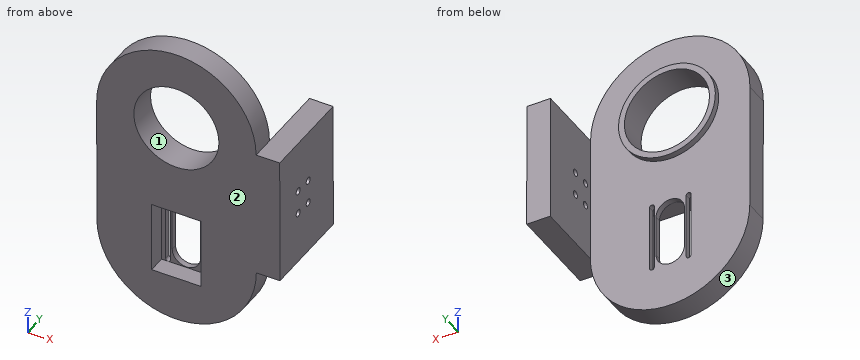
```python
from build123d import *

# Parameters (mm, degrees)
BOSS_EXTRUDE1_DEPTH = 20
SKETCH8_W           = 42
SKETCH8_H           = 60
CUT_EXTRUDE1_DEPTH  = 15
CUT_EXTRUDE2_START  = -5
CUT_EXTRUDE2_DEPTH  = 5
SKETCH10_R          = 36
CUT_EXTRUDE3_DEPTH  = 159.272933389
SKETCH11_R          = 41
SKETCH11_R_2        = 36
BOSS_EXTRUDE4_DEPTH = 5
SKETCH2_W           = 108.361469825
SKETCH2_H           = 80
SKETCH2_R           = 3
BOSS_EXTRUDE6_DEPTH = 20


# Read off the part's stored shape, not the designer's step: Cut-Extrude2
with BuildPart() as part:
    # Sketch1 → Boss-Extrude1 (new body)
    with BuildSketch(Plane(origin=(0, 0, 0), x_dir=(1, 0, 0), z_dir=(0, 1, 0))):
        with BuildLine():
            Line((47.685345344, 62.745795153), (47.499901156, -45.615515992))
            ThreePointArc((47.499901156, -45.615515992), (-20.115515992, -112.999901156), (-87.499901156, -45.384484008))
            Line((-87.499901156, -45.384484008), (-87.314456968, 62.976827137))
            ThreePointArc((-87.314456968, 62.976827137), (-19.69903982, 130.361212301), (47.685345344, 62.745795153))
        make_face()
    extrude(amount=BOSS_EXTRUDE1_DEPTH)

    # Sketch8 → Cut-Extrude1 (cut)
    with BuildSketch(Plane.XZ):
        with Locations((-20, -62.5)):
            Rectangle(SKETCH8_W, SKETCH8_H)
    extrude(amount=-CUT_EXTRUDE1_DEPTH, mode=Mode.SUBTRACT)

    # Cut-Extrude2 outline → Cut-Extrude2 (cut)
    with BuildSketch(Plane.XZ.offset(-15).offset(CUT_EXTRUDE2_START)):
        with BuildLine():
            Line((-6.5, -34.5), (-6.5, -90.5))
            ThreePointArc((-6.5, -90.5), (-4.5, -92.5), (-2.5, -90.5))
            Line((-2.5, -90.5), (-2.5, -34.5))
            ThreePointArc((-2.5, -34.5), (-4.5, -32.5), (-6.5, -34.5))
        make_face()
        with BuildLine():
            ThreePointArc((-8, -45), (-20, -33), (-32, -45))
            Line((-32, -45), (-32, -80))
            ThreePointArc((-32, -80), (-20, -92), (-8, -80))
            Line((-8, -80), (-8, -45))
        make_face()
        with BuildLine():
            Line((-37.5, -34.5), (-37.5, -90.5))
            ThreePointArc((-37.5, -90.5), (-35.5, -92.5), (-33.5, -90.5))
            Line((-33.5, -90.5), (-33.5, -34.5))
            ThreePointArc((-33.5, -34.5), (-35.5, -32.5), (-37.5, -34.5))
        make_face()
    extrude(amount=CUT_EXTRUDE2_DEPTH, mode=Mode.SUBTRACT)

    # Sketch10 → Cut-Extrude3 (cut, through all)
    with BuildSketch(Plane.XZ):
        with Locations(Location((-20, 45.5, 0), (0, 0, 270))):
            Circle(SKETCH10_R)
    extrude(amount=-CUT_EXTRUDE3_DEPTH, mode=Mode.SUBTRACT)

    # Sketch11 → Boss-Extrude4 (add)
    with BuildSketch(Plane(origin=(0, 20, 0), x_dir=(1, 0, 0), z_dir=(0, 1, 0))):
        with Locations(Location((-20, -45.5, 0), (0, 0, 270))):
            Circle(SKETCH11_R)
        with Locations(Location((-20, -45.5, 0), (0, 0, 90))):
            Circle(SKETCH11_R_2, mode=Mode.SUBTRACT)
    extrude(amount=BOSS_EXTRUDE4_DEPTH)

    # Sketch2 → Boss-Extrude6 (add)
    with BuildSketch(Plane(origin=(47.577825951, 0, 0.081422338), x_dir=(0.0017113480294572096, 0, -0.9999985356428889), z_dir=(0.999998535642889, 0, 0.0017113480294572096))):
        with Locations((8.64657458, 40)):
            Rectangle(SKETCH2_W, SKETCH2_H)
        with Locations((-1.551375347, 27.5)):
            Circle(SKETCH2_R, mode=Mode.SUBTRACT)
        with Locations((18.448624653, 27.5)):
            Circle(SKETCH2_R, mode=Mode.SUBTRACT)
        with Locations((18.448624653, 42.5)):
            Circle(SKETCH2_R, mode=Mode.SUBTRACT)
        with Locations((-1.551375347, 42.5)):
            Circle(SKETCH2_R, mode=Mode.SUBTRACT)
    extrude(amount=BOSS_EXTRUDE6_DEPTH)


solid = part.part
```
Could you check a few things on this model? Use its own coordinates, in mm. Face numbers are marked on the shaded views. Coordinates: 2 decimals unless noted, no trailing zeros. Order: outer loops, then holes, each group sorted by start corner. A loop starts at its lowest first (then second) coordinate and runs counter-clockwise, first axis right, second up. Notation, with made-up numbers: M 37.5,-22 L 81.5,-22 A6 cw 81.5,-16 Z; hole C 76.25,25 d2. An arc over 180 degrees is marked long. Use one line per item in the form item = value. Start each with the question number.
1. Please list where these lines run through material, in increasing order: line 1 (Z direction, x = -20, y = 11); line 2 (Z direction, x = 57, y = 28); line 3 (X direction, y = 15, z = 45).
2. We'd pull the mould along X, two halves only. Please class the marked faces 1, 2 and 3: +X half, -X half, draft (parallel to the pull), parting line (faces both ways), or undercut.
3. Suppose I cut it at A-A on z = 22. Write out the boundary of the cut face in (x, y), then the cut area to 3 significant figures.
4. Suppose I cut it at B-B on x = 10. Write out the boundary of the cut face in (y, z).
5. For pin 1 (12 mm diameter, centred on y = 4.5, z = -63, fed in from -X); pin 2 (4 mm diameter, centred on y = 17.5, z = -69.5, fed in from +X); pin 3 (3 mm diameter, centred on x = -2.5, z = -62.5, fed in from -Y), each with a flat end and sliding along its axis, tell me the tip position at first contact or that it passes through.
6. Suppose I cut it at C-C on z = -70.5. Write out the boundary of the cut face in (x, y).
7. Suppose I cut it at D-D on y = 69.5. Write out the boundary of the cut face in (x, z).
Geometry says:
q1.line_1 = -130.36 to -92.5, -32.5 to 9.5, 81.5 to 113
q1.line_2 = -62.73 to -21.31, -15.39 to -1.31, 4.61 to 45.63
q1.line_3 = -87.5 to -56, 16 to 67.5
q2.face_1 = undercut
q2.face_2 = draft
q2.face_3 = parting line
q3.outline = M -87.46,0 L -47.27,0 L -47.27,25 L -53.6,25 L -53.6,20 L -87.46,20 Z; M 7.27,0 L 67.54,0 L 67.54,80 L 47.54,80 L 47.54,20 L 13.6,20 L 13.6,25 L 7.27,25 Z
q3.area = 3,270 mm^2
q4.outline = M 0,-123.42 L 20,-123.42 L 20,17.55 L 25,17.55 L 25,25.6 L 0,25.6 Z; M 0,65.4 L 25,65.4 L 25,73.45 L 20,73.45 L 20,105.97 L 0,105.97 Z
q5.pin_1 = -87.32
q5.pin_2 = 47.53
q5.pin_3 = 15
q6.outline = M -86.88,0 L -41,0 L -41,15 L -37.5,15 L -37.5,20 L -86.88,20 Z; M -33.5,15 L -32,15 L -32,20 L -33.5,20 Z; M -8,15 L -6.5,15 L -6.5,20 L -8,20 Z; M -2.5,15 L 1,15 L 1,0 L 47.25,0 L 47.25,20 L -2.5,20 Z
q7.outline = M 47.5,45.62 L 47.69,-62.75 L 67.69,-62.71 L 67.5,45.65 Z
